The listing builds one solid part. Answer for the finished solid, in the listing's coordinates (mm). A direction names the side the tool comes from. Coordinates: 2 decimals unless noted, no trailing zeros. Order: outer loops, then holes, each group sorted by start corner. A loop starts at its lowest first (then second) coordinate and runs counter-clockwise, first axis right, second up.
from build123d import *

# Parameters (mm, degrees)
BOSS_EXTRUDE1_DEPTH = 38.1
SKETCH2_W           = 25.3238
SKETCH2_H           = 160.690428667
CUT_EXTRUDE1_DEPTH  = 77.2
SKETCH3_W           = 152.130858671
SKETCH3_H           = 6.398804689
BOSS_EXTRUDE2_DEPTH = 38.1
SKETCH4_R           = 5.0000027
CUT_EXTRUDE2_DEPTH  = 39.1


with BuildPart() as part:
    # Sketch1 → Boss-Extrude1 (new body)
    with BuildSketch(Plane(origin=(0, 0, 0), x_dir=(0, 0, -1), z_dir=(1, 0, 0))):
        with BuildLine():
            Line((-76.2, 0), (76.2, 0))
            ThreePointArc((76.2, 0), (0, 76.2), (-76.2, 0))
        make_face()
    extrude(amount=BOSS_EXTRUDE1_DEPTH)

    # Sketch2 → Cut-Extrude1 (cut, through all)
    with BuildSketch(Plane.XZ):
        with Locations((19.0881, -0.10655864)):
            Rectangle(SKETCH2_W, SKETCH2_H)
    extrude(amount=-CUT_EXTRUDE1_DEPTH, mode=Mode.SUBTRACT)

    # Sketch3 → Boss-Extrude2 (add)
    with BuildSketch(Plane(origin=(38.1, 0, 0), x_dir=(0, 0, -1), z_dir=(1, 0, 0))):
        with Locations((-0.134570664, 3.199402345)):
            Rectangle(SKETCH3_W, SKETCH3_H)
    extrude(amount=-BOSS_EXTRUDE2_DEPTH)

    # Sketch4 → Cut-Extrude2 (cut, through all)
    with BuildSketch(Plane(origin=(38.1, 0, 0), x_dir=(0, 0, -1), z_dir=(1, 0, 0))):
        with Locations((0, 63.5)):
            Circle(SKETCH4_R)
        with Locations((21.718279101, 59.67048142)):
            Circle(SKETCH4_R)
        with Locations((40.817013215, 48.643822138)):
            Circle(SKETCH4_R)
        with Locations((54.99261314, 31.75)):
            Circle(SKETCH4_R)
        with Locations((62.535292316, 11.026659282)):
            Circle(SKETCH4_R)
        with Locations((-62.535292316, 11.026659282)):
            Circle(SKETCH4_R)
        with Locations((-54.99261314, 31.75)):
            Circle(SKETCH4_R)
        with Locations((-40.817013215, 48.643822138)):
            Circle(SKETCH4_R)
        with Locations((-21.718279101, 59.67048142)):
            Circle(SKETCH4_R)
    extrude(amount=-CUT_EXTRUDE2_DEPTH, mode=Mode.SUBTRACT)


solid = part.part
1) Section A-A (z = 0) is taken. Give the vertices of the cut face in (x, y), then the cut area to 3 significant figures.
2) Each of these flat-tipped pins is pushed along its axis until it touches: P1, Ø3, axis at x = 19.5, z = -1, coming from the +Y side; P2, Ø20.5, axis at x = 16.5, z = -8, coming from the +Y side; P3, Ø13, axis at y = 48.64, z = -40.82, coming from the -X side; P4, Ø4, axis at x = 30.5, z = -3.5, coming from the +Y side. Where does it stop, or does it pass through?
3) Section C-C (y = 31.75) is taken. Give the vertices of the cut face in (x, z), then the cut area to 3 significant figures.
4) Consider L1, parallel to X at y = 60.5, z = -31; L2, parallel to Z at x = 33, y = 31; L3, parallel to Y at x = 1, z = 0. Determine where each line is inside the solid, lowest interval first.
5) Section B-B (x = 22.5) is taken. Give the vertices of the cut face in (y, z).
6) Determine the mould class of faces 1 (the face through (34.97, 58.62, 1.08)), 2 (the face through (6.426, 33, -1)), 3 (the face through (19, 0, 1)) for opening direction Y: released by +Y, released by -Y, zero draft, split by the parting line, or undercut.
7) Section D-D (x = 4.5) is taken. Give the number of separate pieces and of enclosed holes in the cut face, then the cut area to 3 significant figures.
8) A tool of negligible diameter and unlimited length cuts with its end or side. For faces 4 (the face through (34.97, 56.63, -17.75)), 5 (the face through (19, 3, -75.931)), 6 (the face through (31.75, 33, -1)), from which of +Z, -Z, +X, -X, +Y, -Y can it reach the whole face along a straight path? Write none if from no direction.
Filled sheet:
1. outline: (0, 0) - (38.1, 0) - (38.1, 58.5) - (31.75, 58.5) - (31.75, 6.4) - (6.43, 6.4) - (6.43, 58.5) - (0, 58.5) - close; (0, 68.5) - (6.43, 68.5) - (6.43, 76.2) - (0, 76.2) - close; (31.75, 68.5) - (38.1, 68.5) - (38.1, 76.2) - (31.75, 76.2) - close
1. area: 1,010 mm2
2. P1: stops at y = 6.4
2. P2: stops at y = 75.95
2. P3: stops at x = 0
2. P4: stops at y = 76.18
3. outline: (0, -69.27) - (6.43, -69.27) - (6.43, -59.99) - (0, -59.99) - close; (0, -49.99) - (6.43, -49.99) - (6.43, 49.99) - (0, 49.99) - close; (0, 59.99) - (6.43, 59.99) - (6.43, 69.27) - (0, 69.27) - close; (31.75, -69.27) - (38.1, -69.27) - (38.1, -59.99) - (31.75, -59.99) - close; (31.75, -49.99) - (38.1, -49.99) - (38.1, 49.99) - (31.75, 49.99) - close; (31.75, 59.99) - (38.1, 59.99) - (38.1, 69.27) - (31.75, 69.27) - close
3. area: 1,510 mm2
4. L1: x = 0 to 6.43, 31.75 to 38.1
4. L2: z = -69.61 to -59.94, -50.05 to 50.05, 59.94 to 69.61
4. L3: y = 0 to 58.5, 68.5 to 76.2
5. outline: (0, -75.93) - (6.4, -75.93) - (6.4, -64.43) arc R5 cw to (6.4, -60.64) - (6.4, 60.64) arc R5 cw to (6.4, 64.43) - (6.4, 76.2) - (0, 76.2) - close
6. face 1: undercut
6. face 2: zero draft
6. face 3: released by -Y
7. separate pieces: 1
7. enclosed holes: 9
7. area: 8,410 mm2
8. face 4: +X, -X
8. face 5: -Z, +Y, -Y
8. face 6: +Z, -Z, +Y
